Geometry check sheet. Reference: the model listing, model coordinates, mm. A direction names the side the tool comes from. Coordinates: 2 decimals unless noted, no trailing zeros. Write each loop counter-clockwise with the first axis right and the second up, starting at its lowest first coordinate (ties: lowest second). Pieces come first, ordered by that corner, then holes. Notation, with made-up numbers: M 49.5,-10 L 88.5,-10 A4 ccw 88.5,-4 Z; hole C 25.25,68 d10. An arc over 180 degrees is marked long. Answer as a JSON object with one key per item and string values. Group by question number.
```python
from build123d import *

# Parameters (mm, degrees)
CROQUIS1_W              = 8
CROQUIS1_H              = 10
SALIENTE_EXTRUIR1_DEPTH = 3
CROQUIS2_W              = 7
CROQUIS2_H              = 2
CORTAR_EXTRUIR1_DEPTH   = 9
CROQUIS5_W              = 6
CROQUIS5_H              = 7
SALIENTE_EXTRUIR2_DEPTH = 4
CROQUIS6_W              = 6
CROQUIS6_H              = 1.5
SALIENTE_EXTRUIR3_DEPTH = 3
CORTAR_EXTRUIR2_DEPTH   = 1.5
CORTAR_EXTRUIR3_DEPTH   = 2
CROQUIS9_W              = 3
CROQUIS9_H              = 1.5
SALIENTE_EXTRUIR4_DEPTH = 3
CROQUIS10_W             = 4
CROQUIS10_H             = 2
CORTAR_EXTRUIR4_DEPTH   = 7
SALIENTE_EXTRUIR5_DEPTH = 4


with BuildPart() as part:
    # Croquis1 → Saliente-Extruir1 (new body)
    with BuildSketch(Plane(origin=(0, 0, 0), x_dir=(1, 0, 0), z_dir=(0, 1, 0))):
        Rectangle(CROQUIS1_W, CROQUIS1_H)
    extrude(amount=SALIENTE_EXTRUIR1_DEPTH)

    # Croquis2 → Cortar-Extruir1 (cut, through all)
    with BuildSketch(Plane(origin=(4, 0, 0), x_dir=(0, 0, -1), z_dir=(1, 0, 0))):
        with Locations((0, 1)):
            Rectangle(CROQUIS2_W, CROQUIS2_H)
    extrude(amount=-CORTAR_EXTRUIR1_DEPTH, mode=Mode.SUBTRACT)

    # Croquis5 → Saliente-Extruir2 (add)
    with BuildSketch(Plane(origin=(0, 3, 0), x_dir=(1, 0, 0), z_dir=(0, 1, 0))):
        with Locations((-1, 0)):
            Rectangle(CROQUIS5_W, CROQUIS5_H)
    extrude(amount=SALIENTE_EXTRUIR2_DEPTH)

    # Croquis6 → Saliente-Extruir3 (add)
    with BuildSketch(Plane(origin=(0, 3, 0), x_dir=(1, 0, 0), z_dir=(0, 1, 0))):
        with Locations((-1, -4.25)):
            Rectangle(CROQUIS6_W, CROQUIS6_H)
    extrude(amount=SALIENTE_EXTRUIR3_DEPTH)

    # Croquis7 → Cortar-Extruir2 (cut)
    with BuildSketch(Plane.XY.offset(5)):
        Polygon((2, 3), (-4, 6), (2, 6), align=None)
    extrude(amount=-CORTAR_EXTRUIR2_DEPTH, mode=Mode.SUBTRACT)

    # Croquis8 → Cortar-Extruir3 (cut)
    with BuildSketch(Plane(origin=(4, 0, 0), x_dir=(0, 0, -1), z_dir=(1, 0, 0))):
        Polygon((-3.5, 3), (-5, 3), (-5, 0), align=None)
    extrude(amount=-CORTAR_EXTRUIR3_DEPTH, mode=Mode.SUBTRACT)

    # Croquis9 → Saliente-Extruir4 (add)
    with BuildSketch(Plane(origin=(0, 3, 0), x_dir=(1, 0, 0), z_dir=(0, 1, 0))):
        with Locations((-2.5, 4.25)):
            Rectangle(CROQUIS9_W, CROQUIS9_H)
    extrude(amount=SALIENTE_EXTRUIR4_DEPTH)

    # Croquis10 → Cortar-Extruir4 (cut, through all)
    with BuildSketch(Plane(origin=(2, 0, 0), x_dir=(0, 0, -1), z_dir=(1, 0, 0))):
        with Locations((0, 6)):
            Rectangle(CROQUIS10_W, CROQUIS10_H)
    extrude(amount=-CORTAR_EXTRUIR4_DEPTH, mode=Mode.SUBTRACT)

    # Croquis11 → Saliente-Extruir5 (add)
    with BuildSketch(Plane.XY.offset(-2)):
        Polygon((2, 5), (-4, 5), (-4, 7), align=None)
    extrude(amount=SALIENTE_EXTRUIR5_DEPTH)


solid = part.part
```
1) Section check D-D (z = 4.25). Record the cut outline in (x, y), then the cut area to 3 significant figures.
2) Section check B-B (y = 1.5). Record the cut outline in (x, z), then the cut area to 3 significant figures.
3) Go/stop test with flat-tipped pins: pin 1 Ø0.8 at (y, z) = (4, -4) entering from +X; pin 2 Ø3 at (y, z) = (5.5, -1) entering from +X; pin 3 Ø1.6 at (x, y) = (-1.5, 6) entering from +Z. Record where each tip stops, or that it passes through.
4) Material ranges on probe 1 along Z at (x, y) = (-3.25, 1.25); probe 2 along Y at (x, z) = (-0.75, 2.5); probe 3 along Y at (x, z) = (2.5, 1.5), recorded low to high. Write a range as [from, to].
5) Draft check along Z on faces 1 (the flat face through (-1, 2, 5)), 2 (the flat face through (-3, 6, -4)), 3 (the flat face through (0, 2, 0)). Enter one of: +Z half, -Z half, draft (parallel to the pull), parting line (faces both ways), or undercut.
6) Section check A-A (x = 2.5). Record the cut outline in (y, z).
7) Set-up check for faces 4 (the flat face through (0, 1, 3.5)), 5 (the flat face through (2, 1.9, 4.4)), 6 (the flat face through (0, 6, 2)): record each of +Z, -Z, +X, -X, +Y, -Y from which the full face is reachable in a straight line by a thin tool's end or side.
8) Section check C-C (y = 4.5). Record the cut outline in (x, z), then the cut area to 3 significant figures.
Entries:
{
 "1": {"outline": "M -4,0 L 4,0 L 4,1.5 L 2,1.5 L 2,3 L -4,6 Z", "area": "30.0 mm^2"},
 "2": {"outline": "M -4,-5 L 4,-5 L 4,-3.5 L -4,-3.5 Z; M -4,3.5 L 4,3.5 L 4,4.25 L 2,4.25 L 2,5 L -4,5 Z", "area": "22.5 mm^2"},
 "3": {"pin 1": "x = -1", "pin 2": "x = 2", "pin 3": "z = 3.5"},
 "4": {"probe 1": "[-5, -3.5], [3.5, 5]", "probe 2": "[2, 7]", "probe 3": "[2, 3]"},
 "5": {"face 1": "+Z half", "face 2": "draft", "face 3": "undercut"},
 "6": {"outline": "M 0,-5 L 3,-5 L 3,3.5 L 0,5 L 0,3.5 L 2,3.5 L 2,-3.5 L 0,-3.5 Z"},
 "7": {"face 4": "+X, -X, -Y", "face 5": "+Z, +X, +Y", "face 6": "+X, +Y"},
 "8": {"outline": "M -4,-5 L -1,-5 L -1,-3.5 L 2,-3.5 L 2,3.5 L -1,3.5 L -1,5 L -4,5 Z", "area": "51.0 mm^2"}
}
